from build123d import *

# Parameters (mm, degrees)
F0_R     = 11.05
F1_DEPTH = 10
F4_D     = 5
F4_DEPTH = 19.5
F4_TIP   = 1.5021515476
F5_R     = 19
F5_R_2   = 1.55
F5_R_3   = 13.5
F6_DEPTH = 3
F9_D     = 5.1


with BuildPart() as f1:
    # F0 (on Top) → F1 (new body)
    with BuildSketch(Plane.XY):
        with BuildLine():
            ThreePointArc((4.633508996, -12.6799288004), (11.063506936, -7.7362015406), (13.5, 0))
            ThreePointArc((13.5, 0), (-7.7362015406, 11.063506936), (-4.633508996, -12.6799288004))
            ThreePointArc((-4.633508996, -12.6799288004), (0, -13.5), (4.633508996, -12.6799288004))
        make_face()
        Circle(F0_R, mode=Mode.SUBTRACT)
    extrude(amount=F1_DEPTH)

    # F4 (one way)
    with BuildSketch(Plane.XZ.offset(9.75)):
        with Locations((0, 5)):
            Circle(F4_D / 2)
    extrude(amount=-F4_DEPTH, mode=Mode.SUBTRACT)
    with Locations(Plane.XZ.offset(9.75)):
        with Locations((0, 5)):
            with Locations((0, 0, -(F4_DEPTH + F4_TIP / 2))):  # 118° drill point
                Cone(0, F4_D / 2, F4_TIP, mode=Mode.SUBTRACT)

    # F5 (on Top) → F6 (join)
    with BuildSketch(Plane.XY):
        Circle(F5_R)
        with Locations((-11.5448845004, -11.5448845004)):
            Circle(F5_R_2, mode=Mode.SUBTRACT)
        with Locations((11.5448845004, -11.5448845004)):
            Circle(F5_R_2, mode=Mode.SUBTRACT)
        with Locations((-11.5448845004, 11.5448845004)):
            Circle(F5_R_2, mode=Mode.SUBTRACT)
        Circle(F5_R_3, mode=Mode.SUBTRACT)
        with Locations((11.5448845004, 11.5448845004)):
            Circle(F5_R_2, mode=Mode.SUBTRACT)
    extrude(amount=F6_DEPTH)

    # F9 (through all)
    with Locations(Plane.XZ.offset(13.65)):
        with Locations((0, 6.0753664002)):
            Hole(F9_D / 2)


solid = f1.part
Read the model definition and answer for the solid it produces. Units are mm, in the model's axes. Round coordinates to 2 decimals unless told otherwise and drop trailing zeros. Loops run counter-clockwise (first coordinate to the right, second up) from the corner with the lowest first, then second, coordinate; pieces in that order, holes last.
Q1. Section D-D on x = -11.5 is taken. Write down the section's boundary in (y, z).
Q2. Section A-A on x = 0 is taken. Write down the section's boundary in (y, z).
Q3. Each of these flat-tipped pins is pushed along its axis until it touches: pin 1 (8 mm diameter, centred on x = 15, y = -4.5, fed in from +Z); pin 2 (3 mm diameter, centred on x = -9.5, z = 4, fed in from +Y); pin 3 (2 mm diameter, centred on x = -6.5, z = 3.5, fed in from +Y); pin 4 (6 mm diameter, centred on x = -15, z = 3.5, fed in from +Y). Where does it stop, or does it pass through?
Q4. Consider probe 1 along Z at (x, y) = (0, -11.3); probe 2 along Y at (x, z) = (12.5, 2.25); probe 3 along Y at (x, z) = (-5, 3.25). Determine where each line is inside the solid, lowest interval first.
Q5. Determine the mould class of faces 1 (the face through (-4.5, 12.9, 3)), 2 (the face through (8, -8, 0)), 3 (the face through (1.88, 12.15, 7.8)) for opening direction Z: released by +Z, released by -Z, zero draft, split by the parting line, or undercut.
Q6. Section B-B on y = 0 is taken. Write down the section's boundary in (x, z), and give its area (3 significant figures).
Output:
1. outline: (-15.12, 0) - (-13.09, 0) - (-13.09, 3) - (-15.12, 3) - close; (-10, 0) - (10, 0) - (10, 3) - (7.07, 3) - (7.07, 10) - (-7.07, 10) - (-7.07, 3) - (-10, 3) - close; (13.09, 0) - (15.12, 0) - (15.12, 3) - (13.09, 3) - close
2. outline: (-19, 0) - (-11.05, 0) - (-11.05, 3.53) - (-13.5, 3.53) - (-13.5, 3) - (-19, 3) - close; (-13.5, 8.63) - (-11.05, 8.63) - (-11.05, 10) - (-13.5, 10) - close; (11.05, 0) - (19, 0) - (19, 3) - (13.5, 3) - (13.5, 3.53) - (11.05, 3.53) - close; (11.05, 8.63) - (13.5, 8.63) - (13.5, 10) - (11.05, 10) - close
3. pin 1: stops at z = 10
3. pin 2: stops at y = 17.05
3. pin 3: stops at y = 18.15
3. pin 4: stops at y = 14.7
4. probe 1: z = 0 to 3.53, 8.63 to 10
4. probe 2: y = -14.31 to -12.77, -10.32 to 10.32, 12.77 to 14.31
4. probe 3: y = -12.54 to -9.85, 9.85 to 12.54
5. face 1: released by +Z
5. face 2: released by -Z
5. face 3: undercut
6. outline: (-19, 0) - (-11.05, 0) - (-11.05, 10) - (-13.5, 10) - (-13.5, 3) - (-19, 3) - close; (11.05, 0) - (19, 0) - (19, 3) - (13.5, 3) - (13.5, 10) - (11.05, 10) - close
6. area: 82.0 mm2
